Read the model definition and answer for the solid it produces. Units are mm, in the model's axes. Face numbers are marked on the shaded views. Coordinates: 2 decimals unless noted, no trailing zeros. Loops run counter-clockwise (first coordinate to the right, second up) from the corner with the lowest first, then second, coordinate; pieces in that order, holes last. Notation, with made-up numbers: (80.5, 40.25) -> (134.5, 40.25) arc R30 cw to (134.5, 62.25) -> close; hole circle Ø7 at (-13.75, 86.25). An arc over 180 degrees is marked (long way). Answer as a JSON object with one key per item and string values. Group by question number.
Q1. The part is cut by section D-D on x = 100.8. Write down the section's boundary in (y, z), and give its area (3 significant figures).
Q2. The part is cut by section C-C on y = -6.75. Write down the section's boundary in (x, z) (3 decimals).
Q3. Determine the mould class of the marked faces 1, 2, 3 and 4 for opening direction Z: released by +Z, released by -Z, zero draft, split by the parting line, or undercut.
Q4. The part is cut by section B-B on z = 79. Write down the section's boundary in (x, y).
Q5. The part is cut by section A-A on x = 115.37. Write down the section's boundary in (y, z).
Q6. Straight lines are drawn through the part: line 1 along Z through (x, y) = (180.8, -8); line 2 along X through (y, z) = (-3.5, 104); line 3 along Z through (x, y) = (115.37, -5.75). For each, find the intervals that lie inside material, in ascending order. Write a range as [from, to].
from build123d import *

# Parameters (mm, degrees)
SKETCH060_R  = 3.571875
PAD060_DEPTH = 50
SKETCH059_R  = 3.571875
PAD059_DEPTH = 33.7
SKETCH058_R  = 6.35
PAD058_DEPTH = 12.7


with BuildPart() as body060:
    # Sketch060 → Pad060 (new body)
    with BuildSketch(Plane.XZ):
        Circle(SKETCH060_R)
    extrude(amount=PAD060_DEPTH)


with BuildPart() as body060_1:
    # Body060 placement: moved
    add(body060.part.moved(Location((66.23, 10, 105.316))))


with BuildPart() as body059:
    # Sketch059 → Pad059 (new body)
    with BuildSketch(Plane.XZ):
        Circle(SKETCH059_R)
    extrude(amount=PAD059_DEPTH)


with BuildPart() as body059_1:
    # Body059 placement: moved
    add(body059.part.moved(Location((15.37, 5, 105.316))))


with BuildPart() as cut050:
    # Sketch058 → Pad058 (new body)
    with BuildSketch(Plane.XZ):
        with BuildLine():
            Line((0, 59.2), (0, 110))
            Line((0, 110), (37.475, 110))
            ThreePointArc((37.475, 110), (50.8, 96.67502), (64.125, 110))
            Line((64.125, 110), (101.6, 110))
            Line((101.6, 110), (101.6, 59.2))
            Line((101.6, 59.2), (0, 59.2))
        make_face()
        with Locations((10.8, 70.00002)):
            Circle(SKETCH058_R, mode=Mode.SUBTRACT)
        with Locations((90.8, 70.00002)):
            Circle(SKETCH058_R, mode=Mode.SUBTRACT)
    extrude(amount=PAD058_DEPTH)


with BuildPart() as cut050_1:
    # Body058 placement: moved
    add(cut050.part.moved(Location((-10, 0, 10))))

    # Cut049: cut Body059
    add(body059_1.part, mode=Mode.SUBTRACT)

    # Cut050: cut Body060
    add(body060_1.part, mode=Mode.SUBTRACT)


with BuildPart() as cut050_2:
    # Cut050 placement: moved
    add(cut050_1.part.moved(Location((100, 0, 0))))


solid = cut050_2.part
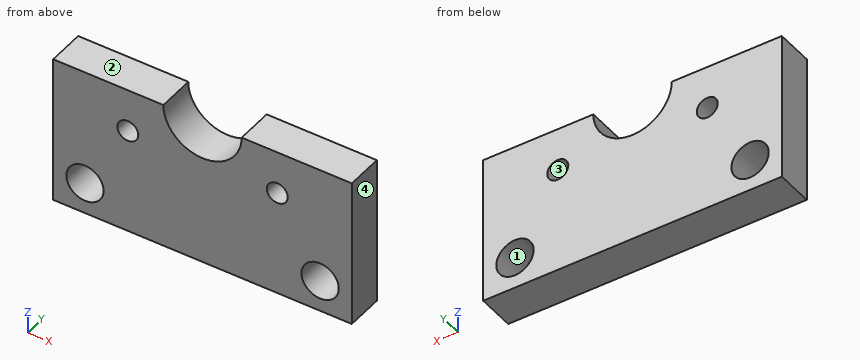
Final values:
{
 "1": {"outline": "(-12.7, 69.2) -> (0, 69.2) -> (0, 73.65) -> (-12.7, 73.65) -> close; (-12.7, 86.35) -> (0, 86.35) -> (0, 120) -> (-12.7, 120) -> close", "area": "484 mm2"},
 "2": {"outline": "(90, 69.2) -> (191.6, 69.2) -> (191.6, 120) -> (154.125, 120) arc R13.325 cw to (127.475, 120) -> (90, 120) -> close; hole circle Ø12.7 at (100.8, 80); hole circle Ø7.144 at (115.37, 105.316); hole circle Ø7.144 at (166.23, 105.316); hole circle Ø12.7 at (180.8, 80)"},
 "3": {"face 1": "undercut", "face 2": "released by +Z", "face 3": "undercut", "face 4": "zero draft"},
 "4": {"outline": "(90, -12.7) -> (94.53, -12.7) -> (94.53, 0) -> (90, 0) -> close; (107.07, -12.7) -> (174.53, -12.7) -> (174.53, 0) -> (107.07, 0) -> close; (187.07, -12.7) -> (191.6, -12.7) -> (191.6, 0) -> (187.07, 0) -> close"},
 "5": {"outline": "(-12.7, 69.2) -> (0, 69.2) -> (0, 101.74) -> (-12.7, 101.74) -> close; (-12.7, 108.89) -> (0, 108.89) -> (0, 120) -> (-12.7, 120) -> close"},
 "6": {"line 1": "z = [69.2, 73.65], [86.35, 120]", "line 2": "x = [90, 112.05], [118.69, 162.91], [169.55, 191.6]", "line 3": "z = [69.2, 101.74], [108.89, 120]"}
}
